Source: CAD feature listing. Evaluate the final solid. Frame: model axes, mm. Round coordinates to 2 decimals unless told otherwise and drop trailing zeros. Write each loop counter-clockwise with the first axis right and the second up, starting at its lowest first coordinate (ties: lowest second). Pieces come first, ordered by that corner, then holes. Notation, with made-up numbers: M 76,36 L 112,36 A23 ccw 112,58 Z; hole C 26,38.5 d1. An arc over 180 degrees is marked long. Answer in a Markdown table with one row per item.
Autodesk Inventor part; units mm, degrees
ref_plane "YZ Plane" through (0, 0, 0) normal (1, 0, 0) x (0, 1, 0)
ref_plane "XZ Plane" through (0, 0, 0) normal (0, 1, 0) x (-1, 0, 0)
ref_plane "XY Plane" through (0, 0, 0) normal (0, 0, 1) x (1, 0, 0)
sketch "Sketch1" plane through (0, 0, 0) normal (0, 0, 1) x (1, 0, 0)
  line L0 (-27, 0) -> (27, 0) construction
  line L1 (-27, -5) -> (27, -5)
  line L2 (27, 5) -> (-27, 5)
  arc A0 (-27, 5) -> (-27, -5) centre (-27, 0) ccw
  arc A1 (27, -5) -> (27, 5) centre (27, 0) ccw
  circle A2 centre (-27, 0) radius 2.1
  circle A3 centre (27, 0) radius 2.1
  point P0 (0, 0)
  point P1 (0, 0)
  point P2 (32, 0)
  dimension "d0" = 5
  dimension "d1" = 4.2
  dimension "d2" = 4.2
  dimension "d3" = 54
extrude "Extrusion1" add sketch "Sketch1" along normal blind 5
properties part number "gate-anchor-link"
Q1. Material intervals for probe 1 along X at (y, z) = (-1.25, 4.8); probe 2 along X at (y, z) = (-0.5, 2.8); probe 3 along Y at (x, z) = (-27, 2.95), sorted ascending.
Solutions:
| item | result |
|---|---|
| probe 1 | x = -31.84 to -28.69, -25.31 to 25.31, 28.69 to 31.84 |
| probe 2 | x = -31.97 to -29.04, -24.96 to 24.96, 29.04 to 31.97 |
| probe 3 | y = -5 to -2.1, 2.1 to 5 |
Q2. Section A-A (y = 0). Return loops of the section in (x, z).
Solutions:
| item | result |
|---|---|
| outline | M -32,0 L -29.1,0 L -29.1,5 L -32,5 Z; M -24.9,0 L 24.9,0 L 24.9,5 L -24.9,5 Z; M 29.1,0 L 32,0 L 32,5 L 29.1,5 Z |
Q3. Pull-direction query (Y, two-part tool) for faces 1 (the flat face through (0, 0, 5)), 2 (the cylindrical face through (-32, 0, 2)), 3 (the cylindrical face through (24.9, -0.09, 2.46)); classes: pulls with the +Y half, pulls with the -Y half, needs draft (parallel to the pull), parting line crosses it, or undercut.
Solutions:
| item | result |
|---|---|
| face 1 | needs draft |
| face 2 | parting line crosses it |
| face 3 | undercut |
Q4. Section C-C (z = 3.9). Return loops of the section in (x, y).
Solutions:
| item | result |
|---|---|
| outline | M -27,-5 L 27,-5 A5 ccw 27,5 L -27,5 A5 ccw Z; hole C -27,0 d4.2; hole C 27,0 d4.2 |
Q5. Contact query for flat-ended pins moving along their axis: pin 1 Ø1 at (y, z) = (3, 3) entering from -X; pin 2 Ø2.5 at (x, y) = (27, 0) entering from +Z. Output: stop coordinate, or through.
Solutions:
| item | result |
|---|---|
| pin 1 | stops at x = -31.33 |
| pin 2 | passes through |
Q6. Section D-D (y = 3.5). Return loops of the section in (x, z).
Solutions:
| item | result |
|---|---|
| outline | M -30.57,0 L 30.57,0 L 30.57,5 L -30.57,5 Z |
Q7. Section B-B (x = -28). Return loops of the section in (y, z), and give its area (3 significant figures).
Solutions:
| item | result |
|---|---|
| outline | M -4.9,0 L -1.85,0 L -1.85,5 L -4.9,5 Z; M 1.85,0 L 4.9,0 L 4.9,5 L 1.85,5 Z |
| area | 30.5 mm2 |
